Source: CAD feature listing. Evaluate the final solid. Frame: model axes, mm. Face numbers are marked on the shaded views. A direction names the side the tool comes from. Coordinates: 2 decimals unless noted, no trailing zeros. Order: outer loops, then holes, each group sorted by start corner. A loop starts at its lowest first (then second) coordinate and runs counter-clockwise, first axis right, second up.
```python
from build123d import *

# Parameters (mm, degrees)
SZKIC1_W                          = 42
SZKIC1_H                          = 42
DODANIE_WYCI_GNI_CIE1_DEPTH       = 9.3
SFAZOWANIE1_SIZE                  = 3.6
ZAOKR_GLENIE1_R                   = 0.5
SZKIC2_W                          = 42
SZKIC2_H                          = 42
DODANIE_WYCI_GNI_CIE2_DEPTH       = 16.7
WYTNIJ_WYCI_GNI_CIE1_DEPTH        = 16.7
ZAOKR_GLENIE2_R                   = 1
SZKIC3_W                          = 42
SZKIC3_H                          = 42
DODANIE_WYCI_GNI_CIE3_DEPTH       = 8
SFAZOWANIE3_SIZE                  = 3.6
ZAOKR_GLENIE3_R                   = 0.5
SZKIC5_R                          = 4.5
WYTNIJ_WYCI_GNI_CIE2_DEPTH        = 4
SZKIC6_R                          = 3
WYTNIJ_WYCI_GNI_CIE3_DEPTH        = 8
SZKIC7_R                          = 1.6
WYTNIJ_WYCI_GNI_CIE4_DEPTH        = 69.439754529
SZKIC20_R                         = 11
DODANIE_WYCI_GNI_CIE4_DEPTH       = 2
ZAOKR_GLENIE4_R                   = 0.5
WYTNIJ_WYCI_GNI_CIE6_START        = -3
SZKIC21_R                         = 4.5
WYTNIJ_WYCI_GNI_CIE6_DEPTH        = 3
DODANIE_WYCI_GNI_CIE5_DEPTH       = 21
SFAZOWANIE4_SIZE                  = 0.5
SZKIC23_W                         = 16
SZKIC23_H                         = 9.3
DODANIE_WYCI_GNI_CIE6_DEPTH       = 4.5
WYTNIJ_WYCI_GNI_CIE7_DEPTH        = 4
SZKIC25_W                         = 0.2
SZKIC25_H                         = 0.2
WYCI_GNI_CIE_CIENKA_CIANKA2_DEPTH = 3
ZAOKR_GLENIE6_R                   = 0.1


with BuildPart() as part:
    # Szkic1 → Dodanie-wyciągnięcie1 (new body)
    with BuildSketch(Plane(origin=(0, 0, 0), x_dir=(1, 0, 0), z_dir=(0, 1, 0))):
        with Locations((21, 21)):
            Rectangle(SZKIC1_W, SZKIC1_H)
    extrude(amount=DODANIE_WYCI_GNI_CIE1_DEPTH)

    # Sfazowanie1
    sfazowanie1_edges = [part.edges().sort_by_distance(p)[0] for p in [
        (0, 4.65, -42),
        (42, 4.65, -42),
        (42, 4.65, 0),
        (0, 4.65, 0),
    ]]
    chamfer(sfazowanie1_edges, length=SFAZOWANIE1_SIZE)

    # Zaokrąglenie1
    zaokr_glenie1_edges = [part.edges().sort_by_distance(p)[0] for p in [
        (0, 4.65, -3.6),
        (0, 4.65, -38.4),
        (38.4, 4.65, -42),
        (3.6, 4.65, -42),
        (38.4, 4.65, 0),
        (3.6, 4.65, 0),
        (42, 4.65, -3.6),
        (42, 4.65, -38.4),
    ]]
    fillet(zaokr_glenie1_edges, radius=ZAOKR_GLENIE1_R)

    # Szkic2 → Dodanie-wyciągnięcie2 (add)
    with BuildSketch(Plane(origin=(0, 9.3, 0), x_dir=(1, 0, 0), z_dir=(0, 1, 0))):
        with Locations((21, 21)):
            Rectangle(SZKIC2_W, SZKIC2_H)
    extrude(amount=DODANIE_WYCI_GNI_CIE2_DEPTH)

    # Szkic4 → Wytnij-wyciągnięcie1 (cut)
    with BuildSketch(Plane(origin=(0, 26, 0), x_dir=(1, 0, 0), z_dir=(0, 1, 0))):
        Polygon((34.928932188, 0), (42, 7.071067812), (42, 0), align=None)
        Polygon((42, 34.928932188), (42, 42), (34.928932188, 42), align=None)
        Polygon((7.071067812, 42), (0, 34.928932188), (0, 42), align=None)
        Polygon((0, 7.071067812), (0, 0), (7.071067812, 0), align=None)
    extrude(amount=-WYTNIJ_WYCI_GNI_CIE1_DEPTH, mode=Mode.SUBTRACT)

    # Zaokrąglenie2
    zaokr_glenie2_edges = [part.edges().sort_by_distance(p)[0] for p in [
        (0, 17.65, -7.071067812),
        (7.071067812, 17.65, 0),
        (7.071067812, 17.65, -42),
        (0, 17.65, -34.928932188),
        (42, 17.65, -34.928932188),
        (34.928932188, 17.65, -42),
        (34.928932188, 17.65, 0),
        (42, 17.65, -7.071067812),
    ]]
    fillet(zaokr_glenie2_edges, radius=ZAOKR_GLENIE2_R)

    # Szkic3 → Dodanie-wyciągnięcie3 (add)
    with BuildSketch(Plane(origin=(0, 26, 0), x_dir=(1, 0, 0), z_dir=(0, 1, 0))):
        with Locations((21, 21)):
            Rectangle(SZKIC3_W, SZKIC3_H)
    extrude(amount=DODANIE_WYCI_GNI_CIE3_DEPTH)

    # Sfazowanie3
    sfazowanie3_edges = [part.edges().sort_by_distance(p)[0] for p in [
        (0, 30, -42),
        (0, 30, 0),
        (42, 30, 0),
        (42, 30, -42),
    ]]
    chamfer(sfazowanie3_edges, length=SFAZOWANIE3_SIZE)

    # Zaokrąglenie3
    zaokr_glenie3_edges = [part.edges().sort_by_distance(p)[0] for p in [
        (38.4, 30, 0),
        (3.6, 30, 0),
        (0, 30, -38.4),
        (0, 30, -3.6),
        (38.4, 30, -42),
        (3.6, 30, -42),
        (42, 30, -38.4),
        (42, 30, -3.6),
    ]]
    fillet(zaokr_glenie3_edges, radius=ZAOKR_GLENIE3_R)

    # Szkic5 → Wytnij-wyciągnięcie2 (cut)
    with BuildSketch(Plane.XZ):
        with Locations(Location((21, -21, 0), (0, 0, 270))):
            Circle(SZKIC5_R)
    extrude(amount=-WYTNIJ_WYCI_GNI_CIE2_DEPTH, mode=Mode.SUBTRACT)

    # Szkic6 → Wytnij-wyciągnięcie3 (cut)
    with BuildSketch(Plane.XZ):
        with Locations(Location((5.6, -5.6, 0), (0, 0, 270))):
            Circle(SZKIC6_R)
        with Locations(Location((36.4, -5.6, 0), (0, 0, 90))):
            Circle(SZKIC6_R)
        with Locations(Location((36.4, -36.4, 0), (0, 0, 270))):
            Circle(SZKIC6_R)
        with Locations(Location((5.6, -36.4, 0), (0, 0, 90))):
            Circle(SZKIC6_R)
    extrude(amount=-WYTNIJ_WYCI_GNI_CIE3_DEPTH, mode=Mode.SUBTRACT)

    # Szkic7 → Wytnij-wyciągnięcie4 (cut, through all)
    with BuildSketch(Plane(origin=(0, 34, 0), x_dir=(1, 0, 0), z_dir=(0, 1, 0))):
        with Locations(Location((36.4, 5.6, 0), (0, 0, 270))):
            Circle(SZKIC7_R)
        with Locations(Location((5.6, 5.6, 0), (0, 0, 90))):
            Circle(SZKIC7_R)
        with Locations(Location((5.6, 36.4, 0), (0, 0, 270))):
            Circle(SZKIC7_R)
        with Locations(Location((36.4, 36.4, 0), (0, 0, 90))):
            Circle(SZKIC7_R)
    extrude(amount=-WYTNIJ_WYCI_GNI_CIE4_DEPTH, mode=Mode.SUBTRACT)

    # Szkic20 → Dodanie-wyciągnięcie4 (add)
    with BuildSketch(Plane(origin=(0, 34, 0), x_dir=(1, 0, 0), z_dir=(0, 1, 0))):
        with Locations(Location((21, 21, 0), (0, 0, 90))):
            Circle(SZKIC20_R)
    extrude(amount=DODANIE_WYCI_GNI_CIE4_DEPTH)

    # Zaokrąglenie4
    zaokr_glenie4_edges = [part.edges().sort_by_distance(p)[0] for p in [
        (21, 34, -10),
    ]]
    fillet(zaokr_glenie4_edges, radius=ZAOKR_GLENIE4_R)

    # Szkic21 → Wytnij-wyciągnięcie6 (cut)
    with BuildSketch(Plane(origin=(0, 36, 0), x_dir=(1, 0, 0), z_dir=(0, 1, 0)).offset(WYTNIJ_WYCI_GNI_CIE6_START)):
        with Locations(Location((21, 21, 0), (0, 0, 90))):
            Circle(SZKIC21_R)
    extrude(amount=WYTNIJ_WYCI_GNI_CIE6_DEPTH, mode=Mode.SUBTRACT)

    # Szkic22 → Dodanie-wyciągnięcie5 (add)
    with BuildSketch(Plane(origin=(0, 33, 0), x_dir=(1, 0, 0), z_dir=(0, 1, 0))):
        with BuildLine():
            Line((19.1, 19.375192319), (19.1, 22.624807681))
            ThreePointArc((19.1, 22.624807681), (23.5, 21), (19.1, 19.375192319))
        make_face()
    extrude(amount=DODANIE_WYCI_GNI_CIE5_DEPTH)

    # Sfazowanie4
    sfazowanie4_edges = [part.edges().sort_by_distance(p)[0] for p in [
        (23.5, 54, -21),
    ]]
    chamfer(sfazowanie4_edges, length=SFAZOWANIE4_SIZE)

    # Szkic23 → Dodanie-wyciągnięcie6 (add)
    with BuildSketch(Plane.XY):
        with Locations((20.992893219, 4.65)):
            Rectangle(SZKIC23_W, SZKIC23_H)
    extrude(amount=DODANIE_WYCI_GNI_CIE6_DEPTH)

    # Szkic24 → Wytnij-wyciągnięcie7 (cut)
    with BuildSketch(Plane.XY.offset(4.5)):
        Polygon((16.592893219, 9.3), (16.592893219, 8.95), (13.892893219, 8.95), (13.892893219, 5.6), (28.092893219, 5.6), (28.092893219, 8.95), (25.392893219, 8.95), (25.392893219, 9.3), align=None)
    extrude(amount=-WYTNIJ_WYCI_GNI_CIE7_DEPTH, mode=Mode.SUBTRACT)

    # Szkic25 → Wyciągnięcie-cienka ścianka2 (add)
    with BuildSketch(Plane.XY.offset(0.5)):
        with Locations((15.892893219, 7.95284256)):
            Rectangle(SZKIC25_W, SZKIC25_H)
        with Locations((17.892893219, 7.95284256)):
            Rectangle(SZKIC25_W, SZKIC25_H)
        with Locations((19.892893219, 7.95284256)):
            Rectangle(SZKIC25_W, SZKIC25_H)
        with Locations((21.892893219, 7.95284256)):
            Rectangle(SZKIC25_W, SZKIC25_H)
        with Locations((23.892893219, 7.95284256)):
            Rectangle(SZKIC25_W, SZKIC25_H)
        with Locations((25.892893219, 7.95284256)):
            Rectangle(SZKIC25_W, SZKIC25_H)
    extrude(amount=WYCI_GNI_CIE_CIENKA_CIANKA2_DEPTH)

    # Zaokrąglenie6
    zaokr_glenie6_edges = [part.edges().sort_by_distance(p)[0] for p in [
        (19.892893219, 7.85284256, 3.5),
        (19.992893219, 7.95284256, 3.5),
        (19.892893219, 8.05284256, 3.5),
        (19.792893219, 7.95284256, 3.5),
        (15.892893219, 7.85284256, 3.5),
        (15.992893219, 7.95284256, 3.5),
        (15.892893219, 8.05284256, 3.5),
        (15.792893219, 7.95284256, 3.5),
        (17.892893219, 7.85284256, 3.5),
        (17.992893219, 7.95284256, 3.5),
        (17.892893219, 8.05284256, 3.5),
        (17.792893219, 7.95284256, 3.5),
        (21.892893219, 7.85284256, 3.5),
        (21.992893219, 7.95284256, 3.5),
        (21.892893219, 8.05284256, 3.5),
        (21.792893219, 7.95284256, 3.5),
        (23.892893219, 7.85284256, 3.5),
        (23.992893219, 7.95284256, 3.5),
        (23.892893219, 8.05284256, 3.5),
        (23.792893219, 7.95284256, 3.5),
        (25.892893219, 7.85284256, 3.5),
        (25.992893219, 7.95284256, 3.5),
        (25.892893219, 8.05284256, 3.5),
        (25.792893219, 7.95284256, 3.5),
    ]]
    fillet(zaokr_glenie6_edges, radius=ZAOKR_GLENIE6_R - 0.0001)  # a hair under: the kernel refuses the full size


solid = part.part
```
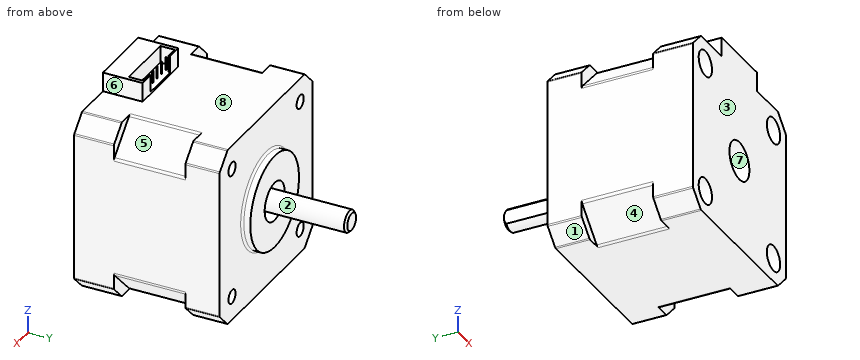
Q1. Pin query (flat end, axial travel): P1, Ø1, axis at x = 18, y = 24, coming from the +Z side; P2, Ø5, axis at x = 7, z = -5, coming from the +Y side; P3, Ø1.5, axis at x = 23, z = -17.5, coming from the +Y side. Return the tip coordinate at first contact, or that it passes through.
Solutions:
P1: stops at z = 0
P2: stops at y = 34
P3: stops at y = 36
Q2. Section query B-B on z = -36.5. Output: boundary loops of the cut face in (x, y), plus the area to 3 significant figures.
Solutions:
outline: (0, 0) - (2.6, 0) - (2.6, 8) - (4, 8) - (4, 34) - (0, 34) - (0, 26) - (1.57, 26) - (1.57, 9.3) - (0, 9.3) - close; (7.2, 8) - (8.6, 8) - (8.6, 0) - (33.4, 0) - (33.4, 8) - (34.8, 8) - (34.8, 34) - (7.2, 34) - close; (38, 8) - (39.4, 8) - (39.4, 0) - (42, 0) - (42, 9.3) - (40.43, 9.3) - (40.43, 26) - (42, 26) - (42, 34) - (38, 34) - close
area: 1,110 mm2
Q3. Material intervals for line 1 along X through (y, z) = (34.45, -21); line 2 along X through (y, z) = (24, -5); line 3 along Z through (x, y) = (5, 19), sorted ascending.
Solutions:
line 1: x = 10 to 16.5, 19.1 to 23.5, 25.5 to 32
line 2: x = 2.07 to 4.12, 7.08 to 34.92, 37.88 to 39.93
line 3: z = -39.93 to -37.88, -34.92 to -7.08, -4.12 to -2.07
Q4. Section query A-A on y = 21. Output: boundary loops of the cut face in (x, z).
Solutions:
outline: (0, -34.51) arc R1 ccw to (0.29, -35.22) - (6.78, -41.71) arc R1 ccw to (7.49, -42) - (34.51, -42) arc R1 ccw to (35.22, -41.71) - (41.71, -35.22) arc R1 ccw to (42, -34.51) - (42, -7.49) arc R1 ccw to (41.71, -6.78) - (35.22, -0.29) arc R1 ccw to (34.51, 0) - (7.49, 0) arc R1 ccw to (6.78, -0.29) - (0.29, -6.78) arc R1 ccw to (0, -7.49) - close; hole circle Ø3.2 at (5.6, -36.4); hole circle Ø3.2 at (5.6, -5.6); hole circle Ø3.2 at (36.4, -36.4); hole circle Ø3.2 at (36.4, -5.6)
Q5. Pull-direction query (X, two-part tool) for the marked faces 6, 7 and 8; classes: pulls with the +X half, pulls with the -X half, needs draft (parallel to the pull), parting line crosses it, or undercut.
Solutions:
face 6: pulls with the +X half
face 7: undercut
face 8: needs draft
Q6. Section query D-D on x = 5.6. Output: boundary loops of the cut face in (y, z).
Solutions:
outline: (0, -42) - (9.3, -42) - (9.3, -40.53) - (26, -40.53) - (26, -42) - (34, -42) - (34, -38) - (8, -38) - (8, -39.4) - (0, -39.4) - close; (0, -33.4) - (8, -33.4) - (8, -34.8) - (34, -34.8) - (34, -7.2) - (8, -7.2) - (8, -8.6) - (0, -8.6) - close; (0, -2.6) - (8, -2.6) - (8, -4) - (34, -4) - (34, 0) - (26, 0) - (26, -1.47) - (9.3, -1.47) - (9.3, 0) - (0, 0) - close
Q7. Section query C-C on x = 21. Output: boundary loops of the cut face in (y, z).
Solutions:
outline: (0, -42) - (34, -42) - (34, -32.5) arc R0.5 cw to (34.5, -32) - (36, -32) - (36, -25.5) - (33, -25.5) - (33, -23.5) - (53.5, -23.5) - (54, -23) - (54, -19) - (53.5, -18.5) - (33, -18.5) - (33, -16.5) - (36, -16.5) - (36, -10) - (34.5, -10) arc R0.5 cw to (34, -9.5) - (34, 0) - (9.3, 0) - (9.3, 0.5) - (5.6, 0.5) - (5.6, 4.5) - (0, 4.5) - (0, -16.5) - (4, -16.5) - (4, -25.5) - (0, -25.5) - close
Q8. Set-up query: the marked faces 1, 2, 3, 4 and 5. Return all of +Z, -Z, +X, -X, +Y, -Y with unobstructed straight access to the full face (end or side cutting, diameter ignored); none if empty.
Solutions:
face 1: -Z, -X, +Y, -Y
face 2: +Y
face 3: +Z, -Z, +X, -X, -Y
face 4: -Z, -X
face 5: +Z, +X
